from build123d import *

# Parameters (mm, degrees)
F1_DEPTH = 3.175


with BuildPart() as f1:
    # F0 (on Right) → F1 (new body)
    with BuildSketch(Plane.YZ):
        Polygon((-40.279892, 18.288), (-40.279892, 0), (-1.5875, 0), (1.5875, 0), (39.935863, 0), (39.935863, 18.288), (1.5875, 18.288), (-1.5875, 18.288), align=None)
        Polygon((-1.5875, 5.08), (-35.199892, 5.08), (-35.199892, 13.208), (-1.5875, 13.208), (1.5875, 13.208), (34.855863, 13.208), (34.855863, 5.08), (1.5875, 5.08), align=None, mode=Mode.SUBTRACT)
    extrude(amount=F1_DEPTH)


solid = f1.part
Could you check a few things on this model? Use its own coordinates, in mm. A direction names the side the tool comes from. Coordinates: 2 decimals unless noted, no trailing zeros. Write each loop counter-clockwise with the first axis right and the second up, starting at its lowest first coordinate (ties: lowest second). Pieces come first, ordered by that corner, then holes. Notation, with made-up numbers: M -27.75,-8 L 29.25,-8 A18 ccw 29.25,0 Z; hole C 80,6 d3. An arc over 180 degrees is marked long. One line per question, with ' | ' between items.
1) If we mould it in two halves opening along Z, with no side actions, what happens to faces 1 (the face through (2, 0, 18.288)), 2 (the face through (2, 0, 5.08)), 3 (the face through (0, -1, 15))? For each: released by +Z, released by -Z, zero draft, split by the parting line, or undercut.
Checks:
face 1: released by +Z | face 2: undercut | face 3: zero draft
2) I need wall thicknesses on probe 1 along Y at (x, z) = (2, 6.25); probe 2 along Z at (x, y) = (1.65, 29.5). Which ranges of each line are inside material? Lowest first, please. Write a range as [from, to].
Checks:
probe 1: [-40.28, -35.2], [34.86, 39.94] | probe 2: [0, 5.08], [13.21, 18.29]
3) For faces 4 (the face through (3.175, -1, 15)), 5 (the face through (2, -1, 13.208)), which set-ups out of +Z, -Z, +X, -X, +Y, -Y let a thin tool reach every point of the face, with its end or its side?
Checks:
face 4: +Z, -Z, +X, +Y, -Y | face 5: +X, -X
4) Imagine slicing it at C-C, the plane y = -12.5. Write out the boundary of the cut face in (x, z) (3 decimals).
Checks:
outline: M 0,0 L 3.175,0 L 3.175,5.08 L 0,5.08 Z; M 0,13.208 L 3.175,13.208 L 3.175,18.288 L 0,18.288 Z
5) Imagine slicing it at B-B, the plane z = 5.75. Write out the boundary of the cut face in (x, y) (3 decimals), and give its area (3 significant figures).
Checks:
outline: M 0,-40.28 L 3.175,-40.28 L 3.175,-35.2 L 0,-35.2 Z; M 0,34.856 L 3.175,34.856 L 3.175,39.936 L 0,39.936 Z | area: 32.3 mm²
6) Imagine slicing it at A-A, the plane x = 0.8. Write out the boundary of the cut face in (y, z).
Checks:
outline: M -40.28,0 L 39.94,0 L 39.94,18.29 L -40.28,18.29 Z; hole M -35.2,5.08 L 34.86,5.08 L 34.86,13.21 L -35.2,13.21 Z
